from build123d import *

# Parameters (mm, degrees)
SKETCH1_W           = 669.8488
SKETCH1_H           = 846.328
BOSS_EXTRUDE1_DEPTH = 19.05
CHAMFER1_SIZE       = 2.54
CHAMFER2_SIZE       = 2.54
CUT_EXTRUDE2_DEPTH  = 670.8488


with BuildPart() as part:
    # Sketch1 → Boss-Extrude1 (new body)
    with BuildSketch(Plane(origin=(0, 0, 0), x_dir=(1, 0, 0), z_dir=(0, 1, 0))):
        with Locations((334.9244, 423.164)):
            Rectangle(SKETCH1_W, SKETCH1_H)
    extrude(amount=BOSS_EXTRUDE1_DEPTH)

    # Chamfer1
    chamfer1_edges = [part.edges().sort_by_distance(p)[0] for p in [
        (669.8488, 19.05, -423.164),
        (334.9244, 19.05, -846.328),
        (0, 19.05, -423.164),
        (334.9244, 19.05, 0),
    ]]
    chamfer(chamfer1_edges, length=CHAMFER1_SIZE)

    # Chamfer2
    chamfer2_edges = [part.edges().sort_by_distance(p)[0] for p in [
        (334.9244, 0, -846.328),
    ]]
    chamfer(chamfer2_edges, length=CHAMFER2_SIZE)

    # Sketch3 → Cut-Extrude2 (cut, through all)
    with BuildSketch(Plane.ZY):
        Polygon((-596.63076, 5.97535), (-596.63076, 0), (-577.58076, 0), (-577.58076, 5.97535), (-574.91376, 5.97535), (-574.91376, 9.53135), (-599.29776, 9.53135), (-599.29776, 5.97535), align=None)
    extrude(amount=-CUT_EXTRUDE2_DEPTH, mode=Mode.SUBTRACT)


solid = part.part
Could you check a few things on this model? Use its own coordinates, in mm. Give positions to 0.01 mm unless a question says otherwise; leave off trailing zeros.
Item 1: I'm going to push a flat-ended pin straight in: pin 1 (7.5 mm diameter, centred on x = 401, z = -589, fed in from -Y). Where does the tip first touch, or does it pass through?
Item 2: I need wall thicknesses on line 1 (Z direction, x = 471, y = 8); line 2 (Z direction, x = 631.5, y = 2.5); line 3 (Z direction, x = 283, y = 16.75). Which ranges of each line are inside material? Lowest first, please.
Item 3: If we mould it in two halves opening along Z, with no side actions, what happens to faces 1 (the face through (330, 8, 0)), 2 (the face through (330, 0, -293)), 3 (the face through (330, 9.531, -587))? For each: pulls with the +Z half, pulls with the -Z half, needs draft (parallel to the pull), parting line crosses it, or undercut.
Values:
1. pin 1: stops at y = 9.53
2. line 1: z = -846.33 to -599.3, -574.91 to 0
2. line 2: z = -846.29 to -596.63, -577.58 to 0
2. line 3: z = -846.09 to -0.24
3. face 1: pulls with the +Z half
3. face 2: needs draft
3. face 3: undercut
